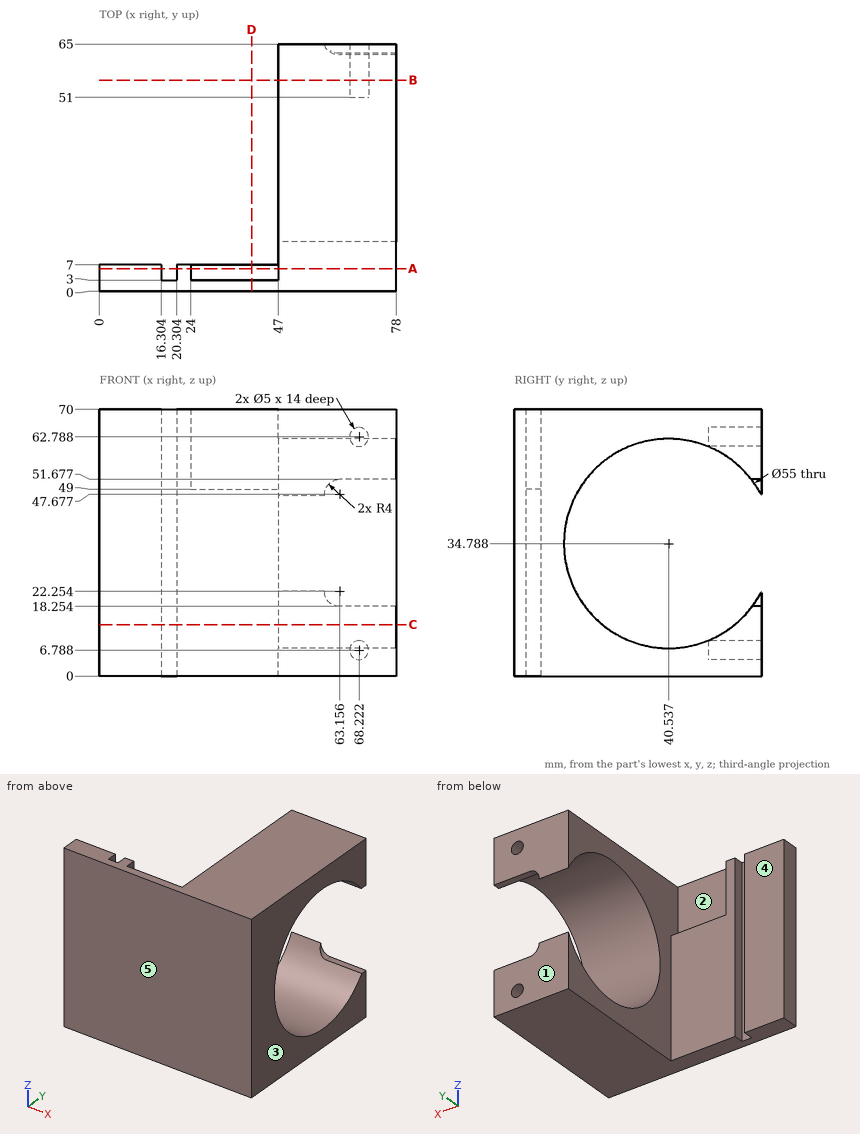
Answer from the drawing. Dimensions are ordinates in mm from the lowest x, y and z of the part. A direction names the side the tool comes from. Give positions to 0.01 mm unless a question says otherwise; leave off trailing zeros. Write each loop counter-clockwise with the first axis right and the second up, starting at its lowest first coordinate (ties: lowest second). Pieces come first, ordered by that corner, then holes.
1) Find the intervals of material crossed by L1, parallel to X at y = 4, z = 35.5 (1 decimal); L2, parallel to Z at x = 49, y = 41.5 (1 decimal); L3, parallel to Y at x = 18.5, z = 42.5, in increasing order.
2) Given P1, Ø23, axis at x = 40, z = 61, coming from the +Y side; P2, Ø4, axis at x = 68.22, z = 6.79, coming from the +Y side; P3, Ø13, axis at x = 8, z = 23.5, coming from the +Y side; P4, Ø3, axis at x = 30, y = 5, coming from the +Z side, each flat-ended and moving along its own axis, determine where each tip first touches the part or whether it passes through.
3) Section D-D (x = 40) is taken. Write down the section's boundary in (y, z).
4) For a pull along X with two mould halves and no side action, classify the marked faces 1, 2 and 3 as pulls with the +X half, pulls with the -X half, needs draft (parallel to the pull), parting line crosses it, or undercut.
5) Section C-C (z = 13.5) is taken. Write down the section's boundary in (x, y) (1 decimal).
6) Section A-A (y = 6) is taken. Write down the section's boundary in (x, z) (1 decimal).
7) A tool of negligible diameter and unlimited length cuts with its end or side. For the marked faces 4 and 5, from which of +Z, -Z, +X, -X, +Y, -Y can it reach the whole face along a straight path? Write none if from no direction.
8) Section B-B (y = 55.5) is taken. Write down the section's boundary in (x, z) (1 decimal), and give its area (3 significant figures).
Response:
1. L1: x = 0 to 16.3, 20.3 to 78
1. L2: z = 0 to 7.3, 62.3 to 70
1. L3: y = 0 to 3
2. P1: stops at y = 65
2. P2: stops at y = 51
2. P3: stops at y = 7
2. P4: stops at z = 49
3. outline: (0, 0) - (7, 0) - (7, 49) - (3, 49) - (3, 70) - (0, 70) - close
4. face 1: needs draft
4. face 2: undercut
4. face 3: pulls with the +X half
5. outline: (0, 0) - (78, 0) - (78, 23.1) - (47, 23.1) - (47, 7) - (20.3, 7) - (20.3, 3) - (16.3, 3) - (16.3, 7) - (0, 7) - close; (47, 57.9) - (78, 57.9) - (78, 65) - (47, 65) - close
6. outline: (0, 0) - (16.3, 0) - (16.3, 70) - (0, 70) - close; (20.3, 0) - (78, 0) - (78, 70) - (47, 70) - (47, 49) - (24, 49) - (24, 70) - (20.3, 70) - close
7. face 4: +Z, -Z, -X, +Y
7. face 5: +Z, -Z, +X, -X, -Y
8. outline: (47, 0) - (78, 0) - (78, 11.7) - (47, 11.7) - close; (47, 57.9) - (78, 57.9) - (78, 70) - (47, 70) - close; hole circle Ø5 at (68.2, 6.8); hole circle Ø5 at (68.2, 62.8)
8. area: 700 mm2
